```python
from build123d import *

# Parameters (mm, degrees)
SKETCH2_R           = 5.1435
BOSS_EXTRUDE1_DEPTH = 12.319
SKETCH3_R           = 2.794
CUT_EXTRUDE1_DEPTH  = 25.638
BOSS_EXTRUDE2_DEPTH = 2.54
SKETCH3_2_R         = 2.794
CUT_EXTRUDE2_DEPTH  = 25.638


with BuildPart() as part:
    # Sketch2 → Boss-Extrude1 (new body, symmetric)
    with BuildSketch(Plane.XY):
        Circle(SKETCH2_R)
    extrude(amount=BOSS_EXTRUDE1_DEPTH, both=True)

    # Sketch3 → Cut-Extrude1 (cut, through all)
    with BuildSketch(Plane.XY.offset(12.319)):
        Circle(SKETCH3_R)
    extrude(amount=-CUT_EXTRUDE1_DEPTH, mode=Mode.SUBTRACT)

    # Sketch4 → Boss-Extrude2 (add, symmetric)
    with BuildSketch(Plane.XY):
        Polygon((3.207902433, 5.55625), (-3.207902433, 5.55625), (-6.415804866, 0), (-3.207902433, -5.55625), (3.207902433, -5.55625), (6.415804866, 0), align=None)
    extrude(amount=BOSS_EXTRUDE2_DEPTH, both=True)

    # Sketch3<2> → Cut-Extrude2 (cut, through all)
    with BuildSketch(Plane.XY.offset(12.319)):
        Circle(SKETCH3_2_R)
    extrude(amount=-CUT_EXTRUDE2_DEPTH, mode=Mode.SUBTRACT)


solid = part.part
```
Source: CAD feature listing. Evaluate the final solid. Frame: model axes, mm. A direction names the side the tool comes from. Coordinates: 2 decimals unless noted, no trailing zeros. Write each loop counter-clockwise with the first axis right and the second up, starting at its lowest first coordinate (ties: lowest second). Pieces come first, ordered by that corner, then holes. Notation, with made-up numbers: (35.5, -30) -> (73.5, -30) arc R7 ccw to (73.5, -25) -> close; hole circle Ø7 at (28, -21.5). An arc over 180 degrees is marked (long way). Return JSON: item names as keys, results as strings. Group by question number.
1) Contact query for flat-ended pins moving along their axis: P1, Ø5, axis at y = -1.5, z = -9.5, coming from the -X side; P2, Ø1, axis at x = -1.5, y = -1, coming from the -Z side; P3, Ø6, axis at x = -2.5, z = -8.5, coming from the +Y side; P4, Ø1, axis at x = -3, z = -5, coming from the +Y side. Output: stop coordinate, or through.
2) Mould query, pull axis X, two halves, no side actions, for faces 4 (the face through (-2.217, -1.7, 0.172)), 5 (the face through (-4.834, -2.739, 0.036)), 6 (the face through (2.2, -2.2, -12.319)). Classes: +X half, -X half, draft (parallel to the pull), parting line (faces both ways), or undercut.
3) Ray query, line 1 along Y through (x, z) = (0, 5); line 2 along Y through (x, z) = (0, 1.25); line 3 along Z through (x, y) = (5.75, 1). Return the intervals inside material, ascending.
4) Section query B-B, the plane z = 2.25. Return loops of the section in (x, y).
5) Section query C-C, the plane y = 2. Return loops of the section in (x, z), plus the area to 3 significant figures.
6) Section query A-A, the plane x = 0. Return loops of the section in (y, z), plus the area to 3 significant figures.
7) Set-up query: faces 1 (the face through (4.834, 2.739, 0.036)), 2 (the face through (-0.67, 5.1, 7.5)), 3 (the face through (-0.67, 5.1, -7.36)). Return all of +Z, -Z, +X, -X, +Y, -Y with unobstructed straight access to the full face (end or side cutting, diameter ignored); none if empty.
8) Section query D-D, the plane x = -4.5. Return loops of the section in (y, z).
From the geometry:
{
 "1": {"P1": "x = -5.14", "P2": "through", "P3": "y = 5.14", "P4": "y = 4.5"},
 "2": {"face 4": "undercut", "face 5": "-X half", "face 6": "draft"},
 "3": {"line 1": "-5.14 to -2.79, 2.79 to 5.14", "line 2": "-5.56 to -2.79, 2.79 to 5.56", "line 3": "-2.54 to 2.54"},
 "4": {"outline": "(-6.42, 0) -> (-3.21, -5.56) -> (3.21, -5.56) -> (6.42, 0) -> (3.21, 5.56) -> (-3.21, 5.56) -> close; hole circle Ø5.59 at (0, 0)"},
 "5": {"outline": "(-5.26, -2.54) -> (-4.74, -2.54) -> (-4.74, -12.32) -> (-1.95, -12.32) -> (-1.95, 12.32) -> (-4.74, 12.32) -> (-4.74, 2.54) -> (-5.26, 2.54) -> close; (1.95, -12.32) -> (4.74, -12.32) -> (4.74, -2.54) -> (5.26, -2.54) -> (5.26, 2.54) -> (4.74, 2.54) -> (4.74, 12.32) -> (1.95, 12.32) -> close", "area": "143 mm²"},
 "6": {"outline": "(-5.56, -2.54) -> (-5.14, -2.54) -> (-5.14, -12.32) -> (-2.79, -12.32) -> (-2.79, 12.32) -> (-5.14, 12.32) -> (-5.14, 2.54) -> (-5.56, 2.54) -> close; (2.79, -12.32) -> (5.14, -12.32) -> (5.14, -2.54) -> (5.56, -2.54) -> (5.56, 2.54) -> (5.14, 2.54) -> (5.14, 12.32) -> (2.79, 12.32) -> close", "area": "120 mm²"},
 "7": {"face 1": "+Z, -Z, +X, +Y", "face 2": "+Z", "face 3": "-Z"},
 "8": {"outline": "(-3.32, -2.54) -> (-2.49, -2.54) -> (-2.49, -12.32) -> (2.49, -12.32) -> (2.49, -2.54) -> (3.32, -2.54) -> (3.32, 2.54) -> (2.49, 2.54) -> (2.49, 12.32) -> (-2.49, 12.32) -> (-2.49, 2.54) -> (-3.32, 2.54) -> close"}
}
